from build123d import *

# Parameters (mm, degrees)
SKETCH_1_R      = 5
SKETCH_1_R_2    = 3.07
EXTRUDE_1_DEPTH = 5
SKETCH_2_W      = 11.338543919
SKETCH_2_H      = 3.370146556
EXTRUDE_2_DEPTH = 7
SKETCH_3_R      = 1.58
EXTRUDE_3_DEPTH = 6


with BuildPart() as part:
    # Sketch 1 → Extrude 1 (new body)
    with BuildSketch(Plane(origin=(0, 0, 0), x_dir=(1, 0, 0), z_dir=(0, 1, 0))):
        with Locations(Location((0, 0.826021493, 0), (0, 0, 270))):
            Circle(SKETCH_1_R)
        with Locations(Location((0, 0.826021493, 0), (0, 0, 270))):
            Circle(SKETCH_1_R_2, mode=Mode.SUBTRACT)
    extrude(amount=EXTRUDE_1_DEPTH)


with BuildPart() as body_2:
    # Sketch 2 → Extrude 2 (new body)
    with BuildSketch(Plane(origin=(0, 5, 0), x_dir=(1, 0, 0), z_dir=(0, 1, 0))):
        with Locations((-0.160637922, 0.629667615)):
            Rectangle(SKETCH_2_W, SKETCH_2_H)
    extrude(amount=-EXTRUDE_2_DEPTH)


with BuildPart() as body_3:
    # Sketch 3 → Extrude 3 (new body)
    with BuildSketch(Plane(origin=(5.508634037, 0, 0), x_dir=(0, 0, -1), z_dir=(1, 0, 0))):
        with Locations((0.826021493, 2.5)):
            Circle(SKETCH_3_R)
    extrude(amount=-EXTRUDE_3_DEPTH)


with BuildPart() as part_1:
    add(part.part)

    # Combine 1: cut body 3
    add(body_3.part, mode=Mode.SUBTRACT)


solid = part_1.part
Design review of the part built by this model. Coordinates are the model's own, in mm. Round coordinates to 2 decimals unless told otherwise and drop trailing zeros. Write each loop counter-clockwise with the first axis right and the second up, starting at its lowest first coordinate (ties: lowest second). Pieces come first, ordered by that corner, then holes.
Item 1: For pin 1 Ø1 at (x, y) = (2, 2) entering from +Z; pin 2 Ø1 at (x, y) = (3.5, 2) entering from +Z; pin 3 Ø2 at (x, z) = (0, -2) entering from +Y, all flat-tipped, find the tip position at first contact; note any pin that passes through.
Item 2: Consider section B-B on z = -1.25. Give the boundary of the cut face in (x, y).
Item 3: Consider section C-C on z = -3.5. Give the boundary of the cut face in (x, y).
Item 4: Consider section A-A on x = 0. Give the boundary of the cut face in (y, z), and give its area (3 significant figures).
Item 5: Wall thickness on L1, parallel to Y at x = 3.25, z = -0.75; L2, parallel to Z at x = 2.25, y = 4.8; L3, parallel to X at y = 4.2, z = -3.25: over which ranges is each line inside the solid? List them lowest first.
Item 6: Draft analysis for pull direction Z (two halves, no side actions). For faces 1 (the cylindrical face through (-4.88, 2.46, -1.91)), 2 (the flat face through (-3.3, 5, -0.9)), 3 (the cylindrical face through (-2.997, 2.465, -1.492)), 4 (the cylindrical face through (3.836, 1.895, -2.286)), state which applies: released by +Z, released by -Z, zero draft, split by the parting line, or undercut.
Item 7: Consider section D-D on y = 4.25. Give the boundary of the cut face in (x, z).
Check values:
1. pin 1: stops at z = 3.94
1. pin 2: stops at z = 3.17
1. pin 3: passes through
2. outline: (-4.98, 0) - (-3.04, 0) - (-3.04, 5) - (-4.98, 5) - close; (3.04, 0) - (4.98, 0) - (4.98, 0.98) - (3.04, 0.98) - close; (3.04, 4.02) - (4.98, 4.02) - (4.98, 5) - (3.04, 5) - close
3. outline: (-4.22, 0) - (-1.51, 0) - (-1.51, 5) - (-4.22, 5) - close; (1.51, 0) - (4.22, 0) - (4.22, 5) - (1.51, 5) - close
4. outline: (0, -5.83) - (5, -5.83) - (5, -3.9) - (0, -3.9) - close; (0, 2.24) - (5, 2.24) - (5, 4.17) - (0, 4.17) - close
4. area: 19.3 mm2
5. L1: y = 0 to 0.92, 4.08 to 5
5. L2: z = -5.29 to -2.91, 1.26 to 3.64
5. L3: x = -4.37 to -1.88, 1.88 to 4.37
6. face 1: split by the parting line
6. face 2: zero draft
6. face 3: undercut
6. face 4: undercut
7. outline: circle Ø10 at (0, -0.83); hole circle Ø6.14 at (0, -0.83)
